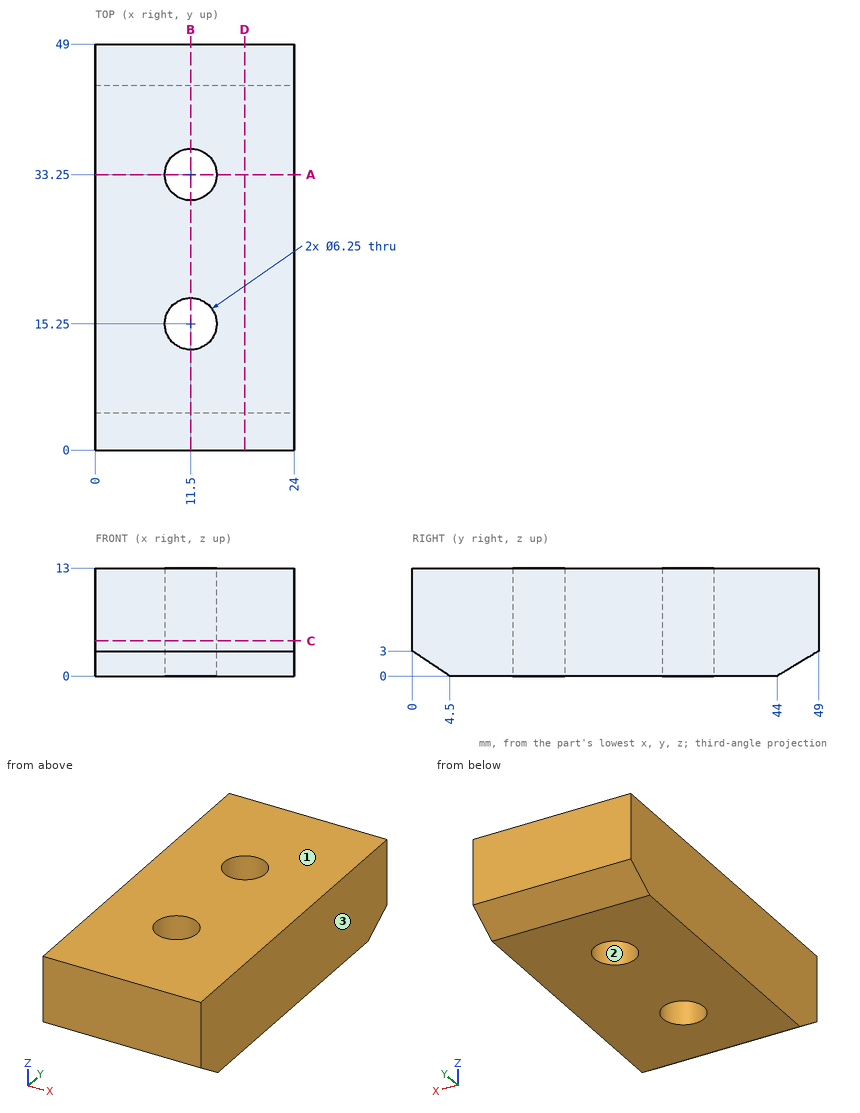
Can you work these out from the drawing? Everything is in mm from the part's minimum corner. Coordinates: 2 decimals unless noted, no trailing zeros. Write each loop counter-clockwise with the first axis right and the second up, starting at its lowest first coordinate (ties: lowest second). Pieces come first, ordered by that corner, then holes. Notation, with made-up numbers: (79, -21) -> (115, -21) arc R27 cw to (115, 11) -> close; hole circle Ø8 at (-31.5, 18.5). An arc over 180 degrees is marked (long way). Return JSON: item names as keys, results as strings.
(1) Imagine slicing it at A-A, the plane y = 33.25. Please give me the cut outline in (x, z) (3 decimals).
Numbers:
{"outline": "(0, 0) -> (8.375, 0) -> (8.375, 13) -> (0, 13) -> close; (14.625, 0) -> (24, 0) -> (24, 13) -> (14.625, 13) -> close"}
(2) Imagine slicing it at B-B, the plane x = 11.5. Please give me the cut outline in (y, z) (3 decimals).
Numbers:
{"outline": "(0, 3) -> (4.5, 0) -> (12.125, 0) -> (12.125, 13) -> (0, 13) -> close; (18.375, 0) -> (30.125, 0) -> (30.125, 13) -> (18.375, 13) -> close; (36.375, 0) -> (44, 0) -> (49, 3) -> (49, 13) -> (36.375, 13) -> close"}
(3) Imagine slicing it at D-D, the plane x = 18. Please give me the cut outline in (y, z).
Numbers:
{"outline": "(0, 3) -> (4.5, 0) -> (44, 0) -> (49, 3) -> (49, 13) -> (0, 13) -> close"}
(4) We'd pull the mould along X, two halves only. Please class the marked faces 1, 2 and 3: +X half, -X half, draft (parallel to the pull), parting line (faces both ways), or undercut.
Numbers:
{"face 1": "draft", "face 2": "undercut", "face 3": "+X half"}
(5) I need wall thicknesses on L1, parallel to Y at x = 11.5, z = 8.75 (3 decimals); L2, parallel to X at y = 15.25, z = 9.5 (3 decimals); L3, parallel to Y at x = 10, z = 11.25. Which ranges of each line are inside material? Lowest first, please.
Numbers:
{"L1": "y = 0 to 12.125, 18.375 to 30.125, 36.375 to 49", "L2": "x = 0 to 8.375, 14.625 to 24", "L3": "y = 0 to 12.51, 17.99 to 30.51, 35.99 to 49"}
(6) I'm going to push a flat-ended pin straight in: pin 1 (5.5 mm diameter, centred on x = 11.5, y = 15.25, fed in from -Z). Where does the tip first touch, or does it pass through?
Numbers:
{"pin 1": "passes through"}
(7) Imagine slicing it at C-C, the plane z = 4.25. Please give me the cut outline in (x, y) (3 decimals).
Numbers:
{"outline": "(0, 0) -> (24, 0) -> (24, 49) -> (0, 49) -> close; hole circle Ø6.25 at (11.5, 15.25); hole circle Ø6.25 at (11.5, 33.25)"}
